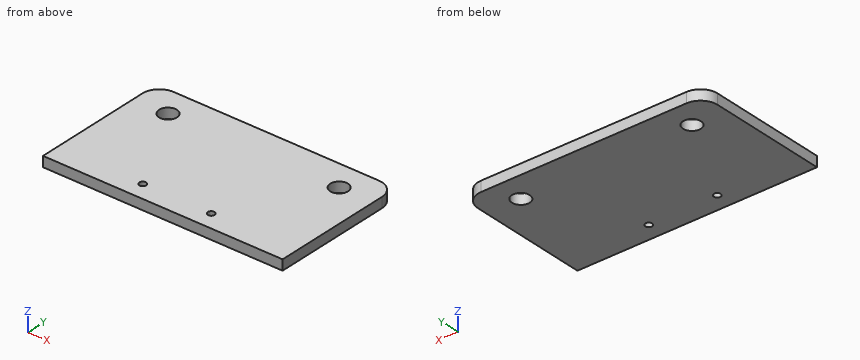
```python
from build123d import *

# Parameters (mm, degrees)
SKETCH_1_R               = 2.6
EXTRUDE_1_DEPTH          = 3
CUT_EXTRUDE_1_DEPTH      = 41.422765863
CUT_EXTRUDE_1_DEPTH_BACK = 41.422765863
SKETCH_2_R               = 1


with BuildPart() as part:
    # Sketch 1 → 凸台-拉伸1 (new body)
    with BuildSketch(Plane.XY):
        with BuildLine():
            Line((-35, -20), (35, -20))
            Line((35, -20), (35, 15))
            ThreePointArc((35, 15), (33.535533906, 18.535533906), (30, 20))
            Line((30, 20), (-30, 20))
            ThreePointArc((-30, 20), (-33.535533906, 18.535533906), (-35, 15))
            Line((-35, 15), (-35, -20))
        make_face()
        with Locations((-25, 12)):
            Circle(SKETCH_1_R, mode=Mode.SUBTRACT)
        with Locations(Location((25, 12, 0), (0, 0, 180))):
            Circle(SKETCH_1_R, mode=Mode.SUBTRACT)
    extrude(amount=EXTRUDE_1_DEPTH)

    # Sketch 2 → 切除-拉伸1 (cut, two sides: drawn at the far end of the back side and taken through both)
    with BuildSketch(Plane(origin=(0, 0, 0), x_dir=(-1, 0, 0), z_dir=(0, 0, -1)).offset(-CUT_EXTRUDE_1_DEPTH_BACK)):
        with Locations((-10, -15)):
            Circle(SKETCH_2_R)
        with Locations((10, -15)):
            Circle(SKETCH_2_R)
    extrude(amount=CUT_EXTRUDE_1_DEPTH + CUT_EXTRUDE_1_DEPTH_BACK, mode=Mode.SUBTRACT)


solid = part.part
```
Design review of the part built by this model. Coordinates are the model's own, in mm. Give positions to 0.01 mm unless a question says otherwise; leave off trailing zeros. Write each loop counter-clockwise with the first axis right and the second up, starting at its lowest first coordinate (ties: lowest second). Pieces come first, ordered by that corner, then holes.
(1) Wall thickness on line 1 along X through (y, z) = (-15, 1.9); line 2 along Y through (x, z) = (-10, 2.15); line 3 along X through (y, z) = (10, 0.4): over which ranges is each line inside the solid? List them lowest first.
Checked values:
line 1: x = -35 to -11, -9 to 9, 11 to 35
line 2: y = -20 to -16, -14 to 20
line 3: x = -35 to -26.66, -23.34 to 23.34, 26.66 to 35
(2) Add section B-B (y = -15). Give the boundary of the cut face in (x, z).
Checked values:
outline: (-35, 0) - (-11, 0) - (-11, 3) - (-35, 3) - close; (-9, 0) - (9, 0) - (9, 3) - (-9, 3) - close; (11, 0) - (35, 0) - (35, 3) - (11, 3) - close
(3) Clearance check with a flat-ended pin moving along its axis: pin 1 Ø3 at (x, y) = (25, 12) entering from +Z. State where the tip first meets the part, or that it passes through.
Checked values:
pin 1: passes through
(4) Add section C-C (z = 1.6). Give the boundary of the cut face in (x, y), and give its area (3 significant figures).
Checked values:
outline: (-35, -20) - (35, -20) - (35, 15) arc R5 ccw to (30, 20) - (-30, 20) arc R5 ccw to (-35, 15) - close; hole circle Ø5.2 at (-25, 12); hole circle Ø2 at (-10, -15); hole circle Ø2 at (10, -15); hole circle Ø5.2 at (25, 12)
area: 2,740 mm2
(5) Add section A-A (x = -10). Give the boundary of the cut face in (y, z), and give its area (3 significant figures).
Checked values:
outline: (-20, 0) - (-16, 0) - (-16, 3) - (-20, 3) - close; (-14, 0) - (20, 0) - (20, 3) - (-14, 3) - close
area: 114 mm2
(6) Add section D-D (x = -25). Give the boundary of the cut face in (y, z).
Checked values:
outline: (-20, 0) - (9.4, 0) - (9.4, 3) - (-20, 3) - close; (14.6, 0) - (20, 0) - (20, 3) - (14.6, 3) - close
